Geometry: final body of the model. Coordinates: model frame, mm. A direction names the side the tool comes from. Give positions to 0.01 mm unless a question says otherwise; leave off trailing zeros. Write each loop counter-clockwise with the first axis right and the second up, starting at its lowest first coordinate (ties: lowest second). Pieces come first, ordered by that corner, then holes. Notation, with made-up numbers: M 24.5,42 L 72.5,42 A12 ccw 72.5,58 Z; hole C 57,34 d5. An arc over 180 degrees is marked long. Answer as a JSON object with one key per item and string values.
from build123d import *

# Parameters (mm, degrees)
F0_R           = 16.5
F1_DEPTH       = 30
F5_D           = 9
F5_START       = 1.5000001
F5_CBORE_D     = 13
F5_CBORE_DEPTH = 9
F8_D           = 13
F8_DEPTH       = 20
F8_START       = 0.8597847
F8_TIP         = 3.9055940237


with BuildPart() as f1:
    # F0 (on Front) → F1 (new body)
    with BuildSketch(Plane.XZ):
        with BuildLine():
            ThreePointArc((-28.2352941176, -22.0588235294), (-18.5626768572, -12.8623938857), (-15, 0))
            ThreePointArc((-15, 0), (-18.5626768572, 12.8623938857), (-28.2352941176, 22.0588235294))
            ThreePointArc((-28.2352941176, 22.0588235294), (-65, 0), (-28.2352941176, -22.0588235294))
        make_face()
        with Locations((-40, 0)):
            Circle(F0_R, mode=Mode.SUBTRACT)
        with BuildLine():
            ThreePointArc((-28.2352941176, 22.0588235294), (-18.5626768572, 12.8623938857), (-15, 0))
            Line((-15, 0), (-15, 15))
            Line((-15, 15), (-28.2352941176, 22.0588235294))
        make_face()
        with BuildLine():
            Line((-28.2352941176, -22.0588235294), (-15, -15))
            Line((-15, -15), (-15, 0))
            ThreePointArc((-15, 0), (-18.5626768572, -12.8623938857), (-28.2352941176, -22.0588235294))
        make_face()
        Polygon((-15, -15), (15, -15), (15, 15), (-15, 15), (-15, 0), align=None)
    extrude(amount=F1_DEPTH)

    # F5 (through all)
    # its depths count from where the whole tool has entered the part; down to there all is cleared
    with Locations(Plane(origin=(-25, 0, 0), x_dir=(0, 1, 0), z_dir=(-1, 0, 0)).offset(-F5_START)):
        with Locations((-15, 0)):
            CounterBoreHole(F5_D / 2, F5_CBORE_D / 2, F5_CBORE_DEPTH)

    # F8
    # its depths count from where the whole tool has entered the part; down to there all is cleared
    with Locations(Plane(origin=(-65, 0, 0), x_dir=(0, 1, 0), z_dir=(-1, 0, 0)).offset(-F8_START)):
        with Locations((-15, 0)):
            Hole(F8_D / 2, depth=F8_DEPTH)
            with Locations((0, 0, -(F8_DEPTH + F8_TIP / 2))):  # 118° drill point
                Cone(0, F8_D / 2, F8_TIP, mode=Mode.SUBTRACT)


solid = f1.part
1) Cut plane D-D on x = -1. Return loops of the section in (y, z).
Geometry check:
{"outline": "M -30,-15 L 0,-15 L 0,15 L -30,15 Z; hole C -15,0 d9"}
2) Cut plane A-A on x = -40. Return loops of the section in (y, z), and give its area (3 significant figures).
Geometry check:
{"outline": "M -30,-25 L 0,-25 L 0,-16.5 L -30,-16.5 Z; M -30,16.5 L 0,16.5 L 0,25 L -30,25 Z", "area": "510 mm2"}
3) Line query: line 1 (Z direction, x = -40, y = -12.5); line 2 (Z direction, x = 5, y = -15); line 3 (Z direction, x = -2, y = -5). Output: solid intervals per line, ascending. Write a range as from..to.
Geometry check:
{"line 1": "z = -25..-16.5, 16.5..25", "line 2": "z = -15..-4.5, 4.5..15", "line 3": "z = -15..15"}
4) Cut plane C-C on y = -26. Return loops of the section in (x, z), and give its area (3 significant figures).
Geometry check:
{"outline": "M -28.24,-22.06 L -15,-15 L 15,-15 L 15,15 L -15,15 L -28.24,22.06 A25 ccw long Z; hole C -40,0 d33", "area": "2,080 mm2"}
5) Pull-direction query (Z, two-part tool) for faces 4 (the flat face through (-21.525, -14.79, 18.48)), 5 (the flat face through (-17, 0, 0)), 6 (the cylindrical face through (-32.39, -14.79, -14.64)); classes: pulls with the +Z half, pulls with the -Z half, needs draft (parallel to the pull), parting line crosses it, or undercut.
Geometry check:
{"face 4": "pulls with the +Z half", "face 5": "needs draft", "face 6": "undercut"}
6) Contact query for flat-ended pins moving along their axis: P1, Ø6.5, axis at y = -14, z = -1, coming from the -X side; P2, Ø4, axis at x = -30.5, y = -11.5, coming from the -Z side; P3, Ø5, axis at x = -2, y = -19, coming from the +Z side. Output: stop coordinate, or through.
Geometry check:
{"P1": "stops at x = -14.5", "P2": "stops at z = -23.85", "P3": "stops at z = 15"}
7) Cut plane B-B on z = 0. Return loops of the section in (x, y), and give its area (3 significant figures).
Geometry check:
{"outline": "M -65,-30 L -56.5,-30 L -56.5,-21.5 L -65,-21.5 Z; M -65,-8.5 L -56.5,-8.5 L -56.5,0 L -65,0 Z; M -23.5,-30 L 15,-30 L 15,-19.5 L -14.5,-19.5 L -14.5,-21.5 L -23.5,-21.5 Z; M -23.5,-8.5 L -14.5,-8.5 L -14.5,-10.5 L 15,-10.5 L 15,0 L -23.5,0 Z", "area": "917 mm2"}
8) Set-up query: faces 1 (the flat face through (0, -15, 15)), 2 (the cylindrical face through (-60.152, -21.494, -0.286)), 3 (the flat face through (0, -15, -15)). Return all of +Z, -Z, +X, -X, +Y, -Y with unobstructed straight access to the full face (end or side cutting, diameter ignored); none if empty.
Geometry check:
{"face 1": "+Z, +X, +Y, -Y", "face 2": "-X", "face 3": "-Z, +X, +Y, -Y"}
